Autodesk Inventor part; units mm, degrees
ref_plane "YZ Plane" through (0, 0, 0) normal (1, 0, 0) x (0, 1, 0)
ref_plane "XZ Plane" through (0, 0, 0) normal (0, 1, 0) x (-1, 0, 0)
ref_plane "XY Plane" through (0, 0, 0) normal (0, 0, 1) x (1, 0, 0)
sketch "スケッチ1" plane through (0, 0, 0) normal (0, 0, 1) x (1, 0, 0)
  line L0 (0, 2.3094) -> (2, 1.1547)
  line L1 (2, 1.1547) -> (2, -1.1547)
  line L2 (2, -1.1547) -> (0, -2.3094)
  line L3 (0, -2.3094) -> (-2, -1.1547)
  line L4 (-2, -1.1547) -> (-2, 1.1547)
  line L5 (-2, 1.1547) -> (0, 2.3094)
  point P0 (0, 0)
  point P1 (0, 0)
  dimension "d0" = 4
extrude "押し出し1" add sketch "スケッチ1" along normal blind 6
sketch "スケッチ2" plane through (0, 0, 6) normal (0, 0, 1) x (1, 0, 0)
  circle A0 centre (0, 0) radius 1
  dimension "d3" = 2
extrude "押し出し2" add sketch "スケッチ2" along normal blind 3
thread "ねじ1"
sketch "スケッチ3" plane through (0, 0, 0) normal (0, 0, -1) x (-1, 0, 0)
  point P0 (0, 0)
hole "穴1" at (0, 0, 0) direction (0, 0, 1) diameter 1.567 depth 4 tip angle 118
properties part number "ジュラコンスペーサー（六角・短間段重ね用）_MS-2006-03E" material "アセタール樹脂、白"
Part model, mm, in its own coordinate system. A direction names the side the tool comes from. Give positions to 0.01 mm unless a question says otherwise; leave off trailing zeros. Order: outer loops, then holes, each group sorted by start corner. A loop starts at its lowest first (then second) coordinate and runs counter-clockwise, first axis right, second up. Notation, with made-up numbers: (0.5, 56) - (27.5, 56) arc R15 cw to (27.5, 84) - close; hole circle Ø11 at (9, 62). An arc over 180 degrees is marked (long way). Use a Markdown table: item, result.
1) Saw through at A-A on z = 3.25. List the corners of the cut face in (x, y).
Checked values:
| item | result |
|---|---|
| outline | (-2, -1.15) - (0, -2.31) - (2, -1.15) - (2, 1.15) - (0, 2.31) - (-2, 1.15) - close; hole circle Ø1.57 at (0, 0) |
2) Saw through at B-B on z = 5.5. List the corners of the cut face in (x, y), plus the area to 3 significant figures.
Checked values:
| item | result |
|---|---|
| outline | (-2, -1.15) - (0, -2.31) - (2, -1.15) - (2, 1.15) - (0, 2.31) - (-2, 1.15) - close |
| area | 13.9 mm² |
3) Two-plate mould, pull along X, no slides. Class faces 4 (the conical face through (-0.13, -0.03, 4.39)), 5 (the flat face through (-2, 0, 3)), 6 (the flat face through (2, 0, 3)): +X half, -X half, draft (parallel to the pull), parting line (faces both ways), or undercut.
Checked values:
| item | result |
|---|---|
| face 4 | undercut |
| face 5 | -X half |
| face 6 | +X half |
4) 3-axis set-ups, long thin cutter, end or side, ignore diameter. For faces 1 (the flat face through (0, 0, 9)), 2 (the cylindrical face through (-0.235, 0.747, 2.028)), 3 (the flat face through (-1, 1, 6)): which of +Z, -Z, +X, -X, +Y, -Y reach the whole face in a straight line?
Checked values:
| item | result |
|---|---|
| face 1 | +Z, +X, -X, +Y, -Y |
| face 2 | -Z |
| face 3 | +Z |
5) Flat gauge pin, fed straight in: P1, Ø1, axis at x = -1.5, y = -0.5, coming from the +Z side. Where does the tip first touch, or does it go through?
Checked values:
| item | result |
|---|---|
| P1 | z = 6 |
6) Saw through at C-C on y = 1.4. List the corners of the cut face in (x, z).
Checked values:
| item | result |
|---|---|
| outline | (-1.58, 0) - (1.58, 0) - (1.58, 6) - (-1.58, 6) - close |
7) Saw through at D-D on x = 1.45. List the corners of the cut face in (y, z), plus the area to 3 significant figures.
Checked values:
| item | result |
|---|---|
| outline | (-1.47, 0) - (1.47, 0) - (1.47, 6) - (-1.47, 6) - close |
| area | 17.7 mm² |
8) Probe L1, parallel to X at y = 0, z = 2.8; L2, parallel to Z at x = 1.2, y = 0.85; L3, parallel to X at y = 2.1, z = 4.25. List the from-to ranges inside material, lowest first. Write a range as from..to.
Checked values:
| item | result |
|---|---|
| L1 | -2..-0.78, 0.78..2 |
| L2 | 0..6 |
| L3 | -0.36..0.36 |
